Autodesk Inventor part; units mm, degrees
ref_plane "YZ Plane" through (0, 0, 0) normal (1, 0, 0) x (0, 1, 0)
ref_plane "XZ Plane" through (0, 0, 0) normal (0, 1, 0) x (-1, 0, 0)
ref_plane "XY Plane" through (0, 0, 0) normal (0, 0, 1) x (1, 0, 0)
sketch "Sketch1" plane through (0, 0, 0) normal (0, 0, 1) x (1, 0, 0)
  line L0 (4.6071, -2.8259) -> (-4.3929, -2.8259)
  line L1 (-4.3929, -2.8259) -> (-4.3929, 3.1741)
  line L2 (-4.3929, 3.1741) -> (4.6071, 3.1741)
  line L3 (4.6071, 3.1741) -> (4.6071, -2.8259)
  point P0 (0, 0)
  dimension "d0" = 9
  dimension "d1" = 6
extrude "Extrusion1" add sketch "Sketch1" along normal blind 53
sketch "Sketch2" plane through (-4.3929, 3.1741, 0) normal (0, 1, 0) x (1, 0, 0)
  line L0 (0, 0) -> (9, 0)
  line L1 (0, 0) -> (0, -53)
  line L2 (9, -53) -> (0, -53)
  line L3 (9, 0) -> (9, -53)
  line L4 (-2.9143, -24.5) -> (15.4572, -24.5)
  line L5 (4.5, -53) -> (4.3929, 0)
  circle A0 centre (4.4828, -44.5) radius 1.75
  circle A1 centre (4.4424, -24.5) radius 1.75
  circle A2 centre (4.402, -4.5001) radius 1.75
  dimension "d4" = 3.5
  dimension "d5" = 40
  dimension "d6" = 8.5
  dimension "d9" = 20
hole "Hole1" at (0.09, 3.1741, 44.5) at (0.0495, 3.1741, 24.5) at (0.0091, 3.1741, 4.5001) direction (0, -1, 0) diameter 3.5 end through all counterbore diameter 6 counterbore depth 3.5
properties part number "slider-rail"
Can you work these out from the model? Positions are in its coordinate system, mm. A direction names the side the tool comes from. Coordinates: 2 decimals unless noted, no trailing zeros. Write each loop counter-clockwise with the first axis right and the second up, starting at its lowest first coordinate (ties: lowest second). Pieces come first, ordered by that corner, then holes. Notation, with made-up numbers: (37, 76) -> (59, 76) arc R24 cw to (59, 86) -> close; hole circle Ø8 at (37, 9.5). An arc over 180 degrees is marked (long way). Write each question's results on one line, items separated by ' | '. Start each with the question number.
Item 1: Please list where these lines run through material, in increasing order: probe 1 along Z at (x, y) = (0.09, 1.25); probe 2 along X at (y, z) = (-0.95, 24.5); probe 3 along X at (y, z) = (2.7, 24).
Item 2: If we section it at C-C, the plane x = 1: Write out the boundary of the cut face in (y, z).
Item 3: If we section it at B-B, the plane y = -0.85: Write out the boundary of the cut face in (x, z).
Item 4: On a 3-axis mill with a long thin cutter (end or side, diameter ignored), from which of +Z, -Z, +X, -X, +Y, -Y can I reach the whole of each face in a straight line? I mean faces 1 (the cylindrical face through (-0.082, 1.4, 21.503)), 2 (the cylindrical face through (1.56, -1.59, 5.31)). Say none if no direction works.
Item 5: I'm going to push a flat-ended pin straight in: P1, Ø4.5, axis at x = 0.01, z = 4.5, coming from the +Y side. Where does the tip first touch, or does it pass through?
Item 6: If we section it at D-D, the plane x = -2.25: Write out the boundary of the cut face in (y, z), and give its area (3 significant figures).
Item 7: If we section it at A-A, the plane z = 44.5: Write out the boundary of the cut face in (x, y).
Item 8: Thinking about a two-plate mould opening in Z: for faces 3 (the cylindrical face through (0.8, -1.6, 46.1)), 4 (the flat face through (0, 0, 53)), 5 (the flat face through (-3, 3.174, 26)), 6 (the flat face through (0, 0, 0)), which applies, released by +Z, released by -Z, zero draft, split by the parting line, or undercut?
Answer block:
1) probe 1: 0 to 1.5, 7.5 to 21.5, 27.5 to 41.5, 47.5 to 53 | probe 2: -4.39 to -1.7, 1.8 to 4.61 | probe 3: -4.39 to -2.91, 3.01 to 4.61
2) outline: (-2.83, 0) -> (3.17, 0) -> (3.17, 1.67) -> (-0.33, 1.67) -> (-0.33, 3.06) -> (-2.83, 3.06) -> close; (-2.83, 5.94) -> (-0.33, 5.94) -> (-0.33, 7.33) -> (3.17, 7.33) -> (3.17, 21.65) -> (-0.33, 21.65) -> (-0.33, 23.03) -> (-2.83, 23.03) -> close; (-2.83, 25.97) -> (-0.33, 25.97) -> (-0.33, 27.35) -> (3.17, 27.35) -> (3.17, 41.64) -> (-0.33, 41.64) -> (-0.33, 43.01) -> (-2.83, 43.01) -> close; (-2.83, 45.99) -> (-0.33, 45.99) -> (-0.33, 47.36) -> (3.17, 47.36) -> (3.17, 53) -> (-2.83, 53) -> close
3) outline: (-4.39, 0) -> (4.61, 0) -> (4.61, 53) -> (-4.39, 53) -> close; hole circle Ø3.5 at (0.01, 4.5); hole circle Ø3.5 at (0.05, 24.5); hole circle Ø3.5 at (0.09, 44.5)
4) face 1: +Y | face 2: +Y, -Y
5) P1: y = -0.33
6) outline: (-2.83, 0) -> (3.17, 0) -> (3.17, 2.53) -> (-0.33, 2.53) -> (-0.33, 6.47) -> (3.17, 6.47) -> (3.17, 22.57) -> (-0.33, 22.57) -> (-0.33, 26.43) -> (3.17, 26.43) -> (3.17, 42.62) -> (-0.33, 42.62) -> (-0.33, 46.38) -> (3.17, 46.38) -> (3.17, 53) -> (-2.83, 53) -> close | area: 278 mm²
7) outline: (-4.39, -2.83) -> (-1.66, -2.83) -> (-1.66, -0.33) -> (-2.91, -0.33) -> (-2.91, 3.17) -> (-4.39, 3.17) -> close; (1.84, -2.83) -> (4.61, -2.83) -> (4.61, 3.17) -> (3.09, 3.17) -> (3.09, -0.33) -> (1.84, -0.33) -> close
8) face 3: undercut | face 4: released by +Z | face 5: zero draft | face 6: released by -Z
